Here's how the part is built. I have some questions about the finished solid (model axes, mm). A direction names the side the tool comes from. Coordinates: 2 decimals unless noted, no trailing zeros.
Item 1: Please list where these lines run through material, in increasing order: line 1 (Y direction, x = 50.1, z = 0) (3 decimals); line 2 (Y direction, x = -34.5, z = -0.5); line 3 (Y direction, x = -24.5, z = 3).
Item 2: If we mould it in two halves opening along Z, with no side actions, what happens to faces 6 (the face through (45.72, 29, 0)), 7 (the face through (0.64, 7.523, -28.04)), 8 (the face through (-50.8, -17, -29)), 9 (the face through (-0.71, -31.92, -11.54))? For each: pulls with the +Z half, pulls with the -Z half, needs draft (parallel to the pull), parting line crosses it, or undercut.
Item 3: For faces 1 (the face through (-50.8, -6, 33)), 2 (the face through (0.64, -7.523, 28.04)), 3 (the face through (45.72, -5, 29)), 4 (the face through (-45.72, -27, -10)), 5 (the face through (-0.71, 17.03, 29.36)), which set-ups out of +Z, -Z, +X, -X, +Y, -Y let a thin tool reach every point of the face, with its end or its side?
Item 4: I'm going to push flat-ended pins straight in: P1, Ø2.5, axis at y = 30, z = 1.5, coming from the +X side; P2, Ø4.5, axis at y = -24, z = -17, coming from the -X side; P3, Ø10, axis at x = 35.5, z = -23, coming from the +Y side. Where does each tip first touch, or does it pass through?
from build123d import *

# Parameters (mm, degrees)
SKETCH1_R               = 25.4
BOSS_EXTRUDE1_DEPTH     = 50.8
SKETCH2_R               = 24.13
SKETCH2_R_2             = 12.7
CUT_EXTRUDE1_DEPTH      = 2.54
SKETCH3_R               = 24.13
SKETCH3_R_2             = 12.7
CUT_EXTRUDE2_DEPTH      = 2.54
SKETCH4_W               = 5.08
SKETCH4_H               = 7.62
BOSS_EXTRUDE2_DEPTH     = 45.72
SKETCH5_W               = 101.6
SKETCH5_H               = 10.16
BOSS_EXTRUDE3_DEPTH     = 1.27
CIRPATTERN1_COUNT       = 18
SKETCH6_R               = 9.525
CUT_EXTRUDE3_DEPTH      = 1
CUT_EXTRUDE3_DEPTH_BACK = 102.6


with BuildPart() as part:
    # Sketch1 → Boss-Extrude1 (new body, symmetric)
    with BuildSketch(Plane(origin=(0, 0, 0), x_dir=(0, 0, -1), z_dir=(1, 0, 0))):
        Circle(SKETCH1_R)
    extrude(amount=BOSS_EXTRUDE1_DEPTH, both=True)

    # Sketch2 → Cut-Extrude1 (cut)
    with BuildSketch(Plane(origin=(50.8, 0, 0), x_dir=(0, 0, -1), z_dir=(1, 0, 0))):
        Circle(SKETCH2_R)
        Circle(SKETCH2_R_2, mode=Mode.SUBTRACT)
    extrude(amount=-CUT_EXTRUDE1_DEPTH, mode=Mode.SUBTRACT)

    # Sketch3 → Cut-Extrude2 (cut)
    with BuildSketch(Plane.ZY.offset(50.8)):
        Circle(SKETCH3_R)
        Circle(SKETCH3_R_2, mode=Mode.SUBTRACT)
    extrude(amount=-CUT_EXTRUDE2_DEPTH, mode=Mode.SUBTRACT)

    # Sketch4 → Boss-Extrude2 (add, symmetric)
    with BuildSketch(Plane(origin=(0, 0, 0), x_dir=(0, 0, -1), z_dir=(1, 0, 0))):
        with Locations((0, 28.861090904)):
            Rectangle(SKETCH4_W, SKETCH4_H)
    boss_extrude2 = extrude(amount=BOSS_EXTRUDE2_DEPTH, both=True)

    # Sketch5 → Boss-Extrude3 (add)
    with BuildSketch(Plane(origin=(0, 32.671090904, 0), x_dir=(1, 0, 0), z_dir=(0, 1, 0))):
        Rectangle(SKETCH5_W, SKETCH5_H)
    boss_extrude3 = extrude(amount=BOSS_EXTRUDE3_DEPTH)

    # CirPattern1: Boss-Extrude2, Boss-Extrude3 ×18 about axis
    cirpattern1_axis = Axis((0, 0, 0), (1, 0, 0))
    for i in range(1, CIRPATTERN1_COUNT):
        add(boss_extrude2.rotate(cirpattern1_axis, i * 360 / CIRPATTERN1_COUNT))
        add(boss_extrude3.rotate(cirpattern1_axis, i * 360 / CIRPATTERN1_COUNT))

    # Sketch6 → Cut-Extrude3 (cut, two sides)
    with BuildSketch(Plane(origin=(50.8, 0, 0), x_dir=(0, 0, -1), z_dir=(1, 0, 0))) as cut_extrude3_sk:
        Circle(SKETCH6_R)
    extrude(amount=CUT_EXTRUDE3_DEPTH, mode=Mode.SUBTRACT)
    extrude(cut_extrude3_sk.sketch, amount=-CUT_EXTRUDE3_DEPTH_BACK, mode=Mode.SUBTRACT)


solid = part.part
Answer:
1. line 1: y = -33.941 to -32.671, -25.4 to -24.13, -12.7 to -9.525, 9.525 to 12.7, 24.13 to 25.4, 32.671 to 33.941
1. line 2: y = -33.94 to -9.51, 9.51 to 33.94
1. line 3: y = -33.94 to -32.67, -25.22 to -9.04, 9.04 to 25.22, 32.67 to 33.94
2. face 6: undercut
2. face 7: undercut
2. face 8: needs draft
2. face 9: pulls with the -Z half
3. face 1: +Z, -Z, -X, +Y, -Y
3. face 2: +X, -X
3. face 3: +X
3. face 4: -X
3. face 5: +Z, +X, -X, +Y
4. P1: stops at x = 45.72
4. P2: stops at x = -45.72
4. P3: stops at y = 29.2
